```python
from build123d import *

# Parameters (mm, degrees)
SKETCH_1_R               = 1.2
SKETCH_1_R_2             = 1.425
EXTRUDE_1_DEPTH          = 2
SKETCH_3_R               = 1.9
CUT_EXTRUDE_2_DEPTH      = 1
EXTRUDE_2_DEPTH          = 2
EXTRUDE_3_DEPTH          = 2
PATTERN_CIRCULAR_1_COUNT = 13
PATTERN_CIRCULAR_1_ANGLE = 84
PATTERN_CIRCULAR_2_COUNT = 2
PATTERN_CIRCULAR_2_ANGLE = 7
SKETCH_1_2_R             = 1.2
CUT_EXTRUDE_3_DEPTH      = 2
CUT_EXTRUDE_4_DEPTH      = 3
CUT_EXTRUDE_4_DEPTH_BACK = 3


with BuildPart() as part:
    # 草图1 → 凸台-拉伸1 (new body, symmetric)
    with BuildSketch(Plane(origin=(0, 0, 0), x_dir=(0, 0, -1), z_dir=(1, 0, 0))):
        with BuildLine():
            Line((0, -3), (20, -3))
            ThreePointArc((20, -3), (22.961615091, -0.478368116), (20.944494821, 2.84744263))
            Line((20.944494821, 2.84744263), (-6.768956495, 12.039975948))
            ThreePointArc((-6.768956495, 12.039975948), (-10.195419033, 10.877714688), (-10.011584646, 7.264170488))
            Line((-10.011584646, 7.264170488), (-2.298133329, -1.928362829))
            ThreePointArc((-2.298133329, -1.928362829), (-1.267854785, -2.718923361), (0, -3))
        make_face()
        Circle(SKETCH_1_R, mode=Mode.SUBTRACT)
        with Locations((20, 0)):
            Circle(SKETCH_1_R_2, mode=Mode.SUBTRACT)
        with Locations((-7.713451316, 9.192533317)):
            Circle(SKETCH_1_R, mode=Mode.SUBTRACT)
    extrude(amount=EXTRUDE_1_DEPTH, both=True)

    # 草图3 → 切除-拉伸2 (cut)
    with BuildSketch(Plane(origin=(2, 0, 0), x_dir=(0, 0, -1), z_dir=(1, 0, 0))):
        with Locations((20, 0)):
            Circle(SKETCH_3_R)
    extrude(amount=-CUT_EXTRUDE_2_DEPTH, mode=Mode.SUBTRACT)

    # 草图4 → 凸台-拉伸2 (add, symmetric)
    with BuildSketch(Plane(origin=(0, 0, 0), x_dir=(0, 0, -1), z_dir=(1, 0, 0))):
        with BuildLine():
            Line((-11.14507328, -7.237695215), (0, 0))
            Line((0, 0), (-10.598385285, 16.960961923))
            ThreePointArc((-10.598385285, 16.960961923), (-19.753766812, 3.128689301), (-15.320888862, -12.855752194))
            Line((-15.320888862, -12.855752194), (-11.14507328, -7.237695215))
        make_face()
    extrude(amount=EXTRUDE_2_DEPTH, both=True)

    # 草图4<3> → 凸台-拉伸3 (add, symmetric)
    with BuildSketch(Plane(origin=(0, 0, 0), x_dir=(0, 0, -1), z_dir=(1, 0, 0))):
        with BuildLine():
            Line((-18.450752495, -11.98205877), (-16.773411359, -10.8927807))
            ThreePointArc((-16.773411359, -10.8927807), (-17.407113919, -9.848471202), (-17.975880926, -8.767422936))
            ThreePointArc((-17.975880926, -8.767422936), (-18.278712452, -10.365080481), (-18.450752495, -11.98205877))
        make_face()
    extrude_3 = extrude(amount=EXTRUDE_3_DEPTH, both=True)

    # 阵列(圆周)1: 凸台-拉伸3 ×13 about axis
    pattern_circular_1_axis = Axis((0, 0, 0), (-1, 0, 0))
    for i in range(1, PATTERN_CIRCULAR_1_COUNT):
        add(extrude_3.rotate(pattern_circular_1_axis, i * PATTERN_CIRCULAR_1_ANGLE / (PATTERN_CIRCULAR_1_COUNT - 1)))

    # 阵列(圆周)2: 凸台-拉伸3 ×2 about axis
    pattern_circular_2_axis = Axis((0, 0, 0), (1, 0, 0))
    for i in range(1, PATTERN_CIRCULAR_2_COUNT):
        add(extrude_3.rotate(pattern_circular_2_axis, i * PATTERN_CIRCULAR_2_ANGLE / (PATTERN_CIRCULAR_2_COUNT - 1)))

    # 草图1<2> → 切除-拉伸3 (cut, symmetric)
    with BuildSketch(Plane(origin=(0, 0, 0), x_dir=(0, 0, -1), z_dir=(1, 0, 0))):
        Circle(SKETCH_1_2_R)
    extrude(amount=CUT_EXTRUDE_3_DEPTH, both=True, mode=Mode.SUBTRACT)

    # 草图5 → 切除-拉伸4 (cut, two sides)
    with BuildSketch(Plane(origin=(0, 0, 0), x_dir=(0, 0, -1), z_dir=(1, 0, 0))) as cut_extrude_4_sk:
        Polygon((4, -3), (10.970443107, -1), (17, -3), align=None)
    extrude(amount=CUT_EXTRUDE_4_DEPTH, mode=Mode.SUBTRACT)
    extrude(cut_extrude_4_sk.sketch, amount=-CUT_EXTRUDE_4_DEPTH_BACK, mode=Mode.SUBTRACT)


solid = part.part
```
Check sheet for the modelled part. Datum: model origin and axes. Units: mm. Round coordinates to 2 decimals unless told otherwise and drop trailing zeros. Order: outer loops, then holes, each group sorted by start corner. A loop starts at its lowest first (then second) coordinate and runs counter-clockwise, first axis right, second up. Notation, with made-up numbers: (-4, -28) -> (20, -28) arc R12 ccw to (20, -13) -> close; hole circle Ø2 at (65, 65.25). An arc over 180 degrees is marked (long way). One line per item, written item: value. Start each with the question number.
Q1. Gauge pin test, flat ends, axial feed: pin 1 Ø1.4 at (y, z) = (0, 0) entering from +X; pin 2 Ø6 at (y, z) = (9, -8) entering from +X; pin 3 Ø1.5 at (x, y) = (-1.5, -2.5) entering from -Z. Record the tip position at first contact, or that the pin passes through.
Q2. Cross-section at A-A (y = 0). Record the boundary of the cut face in (x, z) (3 decimals), and give its area (3 significant figures).
Q3. Cross-section at B-B (x = -0.05). Give the number of separate pieces and of enclosed holes in the cut face, and give its area (3 significant figures).
Q4. Thickness scan on line 1 (Z direction, x = -0.6, y = 0) (3 decimals); line 2 (Y direction, x = 0.7, z = 0); line 3 (Y direction, x = -1.2, z = -20) (3 decimals). Record the ranges inside material, lowest first.
Q5. Cross-section at D-D (y = 4). Record the boundary of the cut face in (x, z), and give its area (3 significant figures).
Q6. Mould release check, pull along Y, two halves, no side actions. Record for faces 1 (the face through (0.028, 12.145, 7.182)), 2 (the face through (0.028, -9.212, 18.887)), 3 (the face through (0.028, -1.986, -13.943)): pulls with the +Y half, pulls with the -Y half, needs draft (parallel to the pull), parting line crosses it, or undercut.
Q7. Cross-section at C-C (z = 10). Record the boundary of the cut face in (x, y), and give its area (3 significant figures).
Completed:
1. pin 1: passes through
1. pin 2: stops at x = 2
1. pin 3: stops at z = -22.44
2. outline: (-2, -23) -> (2, -23) -> (2, -21.9) -> (1, -21.9) -> (1, -21.425) -> (-2, -21.425) -> close; (-2, -18.575) -> (1, -18.575) -> (1, -18.1) -> (2, -18.1) -> (2, -1.2) -> (-2, -1.2) -> close; (-2, 1.2) -> (2, 1.2) -> (2, 20.569) -> (-2, 20.569) -> close
2. area: 152 mm²
3. separate pieces: 1
3. enclosed holes: 2
3. area: 583 mm²
4. line 1: z = -23 to -21.425, -18.575 to -1.2, 1.2 to 20.569
4. line 2: y = -3 to -1.2, 1.2 to 9.79
4. line 3: y = -3 to -1.425, 1.425 to 3.161
5. outline: (-2, -17.47) -> (2, -17.47) -> (2, 21.13) -> (-2, 21.13) -> close
5. area: 154 mm²
6. face 1: pulls with the +Y half
6. face 2: undercut
6. face 3: pulls with the -Y half
7. outline: (-2, -6.49) -> (2, -6.49) -> (2, 16) -> (-2, 16) -> close
7. area: 90.0 mm²
